Design review of the part built by this model. Coordinates are the model's own, in mm. Round coordinates to 2 decimals unless told otherwise and drop trailing zeros. Write each loop counter-clockwise with the first axis right and the second up, starting at its lowest first coordinate (ties: lowest second). Pieces come first, ordered by that corner, then holes. Notation, with made-up numbers: M 64,21 L 77,21 A19 cw 77,36 Z; hole C 54.5,55 d4. An arc over 180 degrees is marked long. Use CSV: the item, a comma, the result in double quotes.
from build123d import *

# Parameters (mm, degrees)
ESQUISSE2_W             = 330
ESQUISSE2_H             = 110
BOSS_EXTRU_1_DEPTH      = 6
ESQUISSE4_W             = 168
ESQUISSE4_H             = 6
ESQUISSE4_W_2           = 6
ESQUISSE4_H_2           = 30
ESQUISSE4_W_3           = 50
ESQUISSE4_H_3           = 22
ESQUISSE4_W_4           = 40
ESQUISSE4_W_5           = 3
ENL_V_MAT_EXTRU_1_DEPTH = 348.902285132
ESQUISSE5_R             = 1.5
ENL_V_MAT_EXTRU_2_DEPTH = 6
ESQUISSE6_R             = 2.995
ESQUISSE6_R_2           = 3
ENL_V_MAT_EXTRU_3_DEPTH = 3


with BuildPart() as part:
    # Esquisse2 → Boss.-Extru.1 (new body)
    with BuildSketch(Plane.XY):
        with Locations((165, 55)):
            Rectangle(ESQUISSE2_W, ESQUISSE2_H)
    extrude(amount=BOSS_EXTRU_1_DEPTH)

    # Esquisse4 → Enlèv. mat.-Extru.1 (cut, through all)
    with BuildSketch(Plane.XY.offset(6)):
        with Locations((140, 107)):
            Rectangle(ESQUISSE4_W, ESQUISSE4_H)
        with Locations((3, 45)):
            Rectangle(ESQUISSE4_W_2, ESQUISSE4_H_2)
        with Locations((305, 99)):
            Rectangle(ESQUISSE4_W_3, ESQUISSE4_H_3)
        with Locations((85, 3)):
            Rectangle(ESQUISSE4_W_4, ESQUISSE4_H)
        with Locations((165, 3)):
            Rectangle(ESQUISSE4_W_4, ESQUISSE4_H)
        with Locations((245, 3)):
            Rectangle(ESQUISSE4_W_4, ESQUISSE4_H)
        with Locations((327, 45)):
            Rectangle(ESQUISSE4_W_2, ESQUISSE4_H_2)
        with Locations((133.5, 56)):
            Rectangle(ESQUISSE4_W_5, ESQUISSE4_H_2)
        with Locations((277, 56.5)):
            Rectangle(ESQUISSE4_W_2, ESQUISSE4_H_2)
    extrude(amount=-ENL_V_MAT_EXTRU_1_DEPTH, mode=Mode.SUBTRACT)

    # Esquisse5 → Enlèv. mat.-Extru.2 (cut)
    with BuildSketch(Plane.XY.offset(6)):
        with Locations((3, 23)):
            Circle(ESQUISSE5_R)
        with Locations((58, 3)):
            Circle(ESQUISSE5_R)
        with Locations((112, 3)):
            Circle(ESQUISSE5_R)
        with Locations((138, 3)):
            Circle(ESQUISSE5_R)
        with Locations((192, 3)):
            Circle(ESQUISSE5_R)
        with Locations((218, 3)):
            Circle(ESQUISSE5_R)
        with Locations((272, 3)):
            Circle(ESQUISSE5_R)
        with Locations((277, 34.5)):
            Circle(ESQUISSE5_R)
        with Locations((277, 78.5)):
            Circle(ESQUISSE5_R)
        with Locations((327, 67)):
            Circle(ESQUISSE5_R)
        with Locations((327, 23)):
            Circle(ESQUISSE5_R)
        with Locations((231, 107)):
            Circle(ESQUISSE5_R)
        with Locations((49, 107)):
            Circle(ESQUISSE5_R)
        with Locations((3, 103)):
            Circle(ESQUISSE5_R)
        with Locations((3, 67)):
            Circle(ESQUISSE5_R)
    extrude(amount=-ENL_V_MAT_EXTRU_2_DEPTH, mode=Mode.SUBTRACT)

    # Esquisse6 → Enlèv. mat.-Extru.3 (cut)
    with BuildSketch(Plane.XY.offset(6)):
        with Locations((3, 67)):
            Circle(ESQUISSE6_R)
        with Locations((3, 23)):
            Circle(ESQUISSE6_R)
        with Locations((3, 103)):
            Circle(ESQUISSE6_R)
        with Locations((49, 107)):
            Circle(ESQUISSE6_R)
        with Locations((231, 107)):
            Circle(ESQUISSE6_R)
        with Locations((277, 78.5)):
            Circle(ESQUISSE6_R_2)
        with Locations((327, 67)):
            Circle(ESQUISSE6_R)
        with Locations((277, 34.5)):
            Circle(ESQUISSE6_R)
        with Locations((327, 23)):
            Circle(ESQUISSE6_R)
        with Locations((272, 3)):
            Circle(ESQUISSE6_R)
        with Locations((218, 3)):
            Circle(ESQUISSE6_R)
        with Locations((192, 3)):
            Circle(ESQUISSE6_R)
        with Locations((138, 3)):
            Circle(ESQUISSE6_R)
        with Locations((112, 3)):
            Circle(ESQUISSE6_R)
        with Locations((58, 3)):
            Circle(ESQUISSE6_R)
    extrude(amount=-ENL_V_MAT_EXTRU_3_DEPTH, mode=Mode.SUBTRACT)


solid = part.part
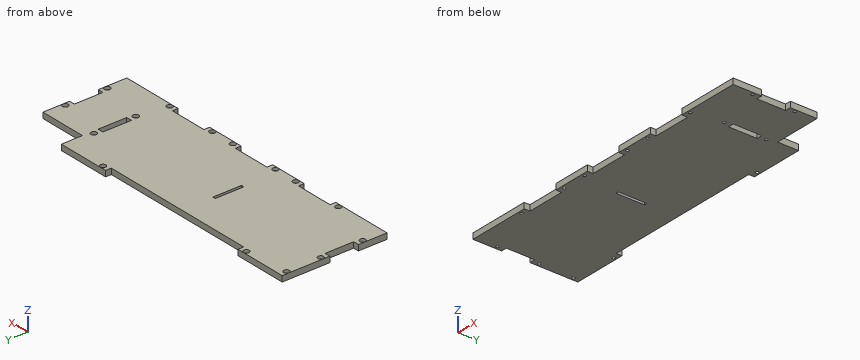
1) Add section B-B on z = 1.4. Give the number of separate pieces and of enclosed holes in the cut face, then the cut area to 3 significant figures.
Answers:
separate pieces,"1"
enclosed holes,"17"
area,"32,700 mm²"
2) For pin 1 Ø1.8 at (x, y) = (3, 67) entering from -Z; pin 2 Ø3 at (x, z) = (254, 1) entering from -Y; pin 3 Ø1.8 at (y, z) = (49, 4) entering from +X; pin 4 Ø3 at (x, y) = (113, 2) entering from +Z, all flat-tipped, find the tip position at first contact; note any pin that passes through.
Answers:
pin 1,"through"
pin 2,"y = 6"
pin 3,"x = 324"
pin 4,"z = 3"
3) Add section A-A on y = 48. Write out the cut boundary in (x, z), then the cut area to 3 significant figures.
Answers:
outline,"M 6,0 L 132,0 L 132,6 L 6,6 Z; M 135,0 L 274,0 L 274,6 L 135,6 Z; M 280,0 L 324,0 L 324,6 L 280,6 Z"
area,"1,850 mm²"
4) Add section C-C on x = 261.5. Write out the cut boundary in (y, z).
Answers:
outline,"M 6,0 L 110,0 L 110,6 L 6,6 Z"
5) Wall thickness on line 1 along X through (y, z) = (50.5, 1.9); line 2 along X through (y, z) = (105, 2.8); line 3 along Y through (x, z) = (3, 5.2) (3 decimals): over which ranges is each line inside the solid? List them lowest first. Write a range as [from, to].
Answers:
line 1,"[6, 132], [135, 274], [280, 324]"
line 2,"[0, 56], [224, 280]"
line 3,"[0, 20.005], [25.995, 30], [60, 64.005], [69.995, 100.005], [105.995, 110]"
6) Add section D-D on x = 83.5. Write out the cut boundary in (y, z), then the cut area to 3 significant figures.
Answers:
outline,"M 6,0 L 104,0 L 104,6 L 6,6 Z"
area,"588 mm²"
